```python
from build123d import *

# Parameters (mm, degrees)
SKETCH1_W           = 320.474741716
SKETCH1_H           = 198.285814429
BOSS_EXTRUDE1_DEPTH = 23.622
SKETCH2_R           = 16.182303952
CUT_EXTRUDE1_DEPTH  = 47.244
LPATTERN1_COUNT     = 5
LPATTERN1_PITCH     = 66.04
LPATTERN1_COL_COUNT = 4
LPATTERN1_COL_PITCH = 45.72


with BuildPart() as part:
    # Sketch1 → Boss-Extrude1 (new, symmetric)
    with BuildSketch(Plane(origin=(0, 0, 0), x_dir=(1, 0, 0), z_dir=(0, 1, 0))):
        with Locations((14.200022321, -53.127541738)):
            Rectangle(SKETCH1_W, SKETCH1_H)
    extrude(amount=BOSS_EXTRUDE1_DEPTH, both=True)

    # Sketch2 → Cut-Extrude1 (cut)
    with BuildSketch(Plane(origin=(0, 23.622, 0), x_dir=(1, 0, 0), z_dir=(0, 1, 0))):
        with Locations(Location((-125.445944565, 26.871307357, 0), (0, 0, 270))):
            Circle(SKETCH2_R)
    cut_extrude1 = extrude(amount=-CUT_EXTRUDE1_DEPTH, mode=Mode.SUBTRACT)

    # LPattern1: Cut-Extrude1 ×5
    with Locations(*[(i * LPATTERN1_PITCH, 0, 0) for i in range(1, LPATTERN1_COUNT)]):
        add(cut_extrude1, mode=Mode.SUBTRACT)

    # LPattern1 col: Cut-Extrude1 ×4
    with Locations(*[(0, 0, i * LPATTERN1_COL_PITCH) for i in range(1, LPATTERN1_COL_COUNT)]):
        add(cut_extrude1, mode=Mode.SUBTRACT)


solid = part.part
```
Design review of the part built by this model. Coordinates are the model's own, in mm. Give positions to 0.01 mm unless a question says otherwise; leave off trailing zeros. Write each loop counter-clockwise with the first axis right and the second up, starting at its lowest first coordinate (ties: lowest second). Pieces come first, ordered by that corner, then holes. Notation, with made-up numbers: (60.25, -2.5) -> (89.25, -2.5) arc R22 ccw to (89.25, 8.5) -> close; hole circle Ø6 at (83, 53.25). An arc over 180 degrees is marked (long way). Answer in a Markdown table with one row per item.
(1) To check wall thickness, follow probe 1 along X at (y, z) = (-20, -25); probe 2 along X at (y, z) = (5, -15); probe 3 along Z at (x, y) = (81.5, 17). State the ranges of each line that lie inside material, in increasing order.
Results:
| item | result |
|---|---|
| probe 1 | -146.04 to -141.52, -109.37 to -75.48, -43.33 to -9.44, 22.71 to 56.6, 88.75 to 122.64, 154.79 to 174.44 |
| probe 2 | -146.04 to -136.44, -114.45 to -70.4, -48.41 to -4.36, 17.63 to 61.68, 83.67 to 127.72, 149.71 to 174.44 |
| probe 3 | -46.02 to -40.43, -13.31 to 152.27 |
(2) Mouldability with a two-part tool opening along X and no side actions: class faces 1 (the cylindrical face through (83.61, 0.33, -38.8)), 2 (the cylindrical face through (-114.51, 0.33, 6.92)), 3 (the flat face through (174.437, 0, 55)), 4 (the flat face through (12, 0, 152.27)) as +X half, -X half, draft (parallel to the pull), parting line (faces both ways), or undercut.
Results:
| item | result |
|---|---|
| face 1 | undercut |
| face 2 | undercut |
| face 3 | +X half |
| face 4 | draft |
(3) Consider section A-A (z = 72). State the section outline as (x, y) points, then the cut area to 3 significant figures.
Results:
| item | result |
|---|---|
| outline | (-146.04, -23.62) -> (-139.82, -23.62) -> (-139.82, 23.62) -> (-146.04, 23.62) -> close; (-111.07, -23.62) -> (174.44, -23.62) -> (174.44, 23.62) -> (-111.07, 23.62) -> close |
| area | 13,800 mm2 |
(4) Consider section B-B (x = 66). State the section outline as (y, z) points.
Results:
| item | result |
|---|---|
| outline | (-23.62, -46.02) -> (23.62, -46.02) -> (23.62, -41.61) -> (-23.62, -41.61) -> close; (-23.62, -12.13) -> (23.62, -12.13) -> (23.62, 152.27) -> (-23.62, 152.27) -> close |
(5) Consider section D-D (y = 19.5). Count the separate pieces of the cut face and the enclosed holes in it, then the cut area to 3 significant figures.
Results:
| item | result |
|---|---|
| separate pieces | 1 |
| enclosed holes | 8 |
| area | 57,000 mm2 |
(6) Consider section C-C (z = -19.5). State the section outline as (x, y) points, then the cut area to 3 significant figures.
Results:
| item | result |
|---|---|
| outline | (-146.04, -23.62) -> (-139.85, -23.62) -> (-139.85, 23.62) -> (-146.04, 23.62) -> close; (-111.04, -23.62) -> (-73.81, -23.62) -> (-73.81, 23.62) -> (-111.04, 23.62) -> close; (-45, -23.62) -> (-7.77, -23.62) -> (-7.77, 23.62) -> (-45, 23.62) -> close; (21.04, -23.62) -> (58.27, -23.62) -> (58.27, 23.62) -> (21.04, 23.62) -> close; (87.08, -23.62) -> (124.31, -23.62) -> (124.31, 23.62) -> (87.08, 23.62) -> close; (153.12, -23.62) -> (174.44, -23.62) -> (174.44, 23.62) -> (153.12, 23.62) -> close |
| area | 8,330 mm2 |
